Verification items for this drawing (mm, ordinates from the low corner). A direction names the side the tool comes from. Round coordinates to 2 decimals unless told otherwise and drop trailing zeros. Write each loop counter-clockwise with the first axis right and the second up, starting at its lowest first coordinate (ties: lowest second). Pieces come first, ordered by that corner, then holes.
Item 1: Cross-section at A-A (x = 29.5). Enter the section's corners in (y, z), then the cut area to 3 significant figures.
Item 2: Cross-section at B-B (y = 6.5). Enter the section's corners in (x, z), then the cut area to 3 significant figures.
Item 3: Access from +Z, -Z, +X, -X, +Y, -Y to the whole of each face (thin tool, end or side, straight path). Record for the marked faces 1, 2 and 3.
Item 4: Scan lines: probe 1 along Y at (x, z) = (4, 27.5) (3 decimals); probe 2 along Z at (x, y) = (8, 0.75); probe 3 along Y at (x, z) = (22, 2). Record each from-to range of solid material in increasing order.
Item 5: Cross-section at C-C (z = 26.5). Enter the section's corners in (x, y) (3 decimals).
Item 6: Cross-section at D-D (x = 9). Enter the section's corners in (y, z).
Item 7: Depth check by flat-ended pin: P1, Ø4, axis at x = 26.5, y = 4.5, coming from the +Z side; P2, Ø1.5, axis at y = 1.5, z = 18.5, coming from the +X side; P3, Ø3, axis at y = 6.5, z = 12.5, coming from the -X side. Enter the tip coordinate at first touch or a pass-through.
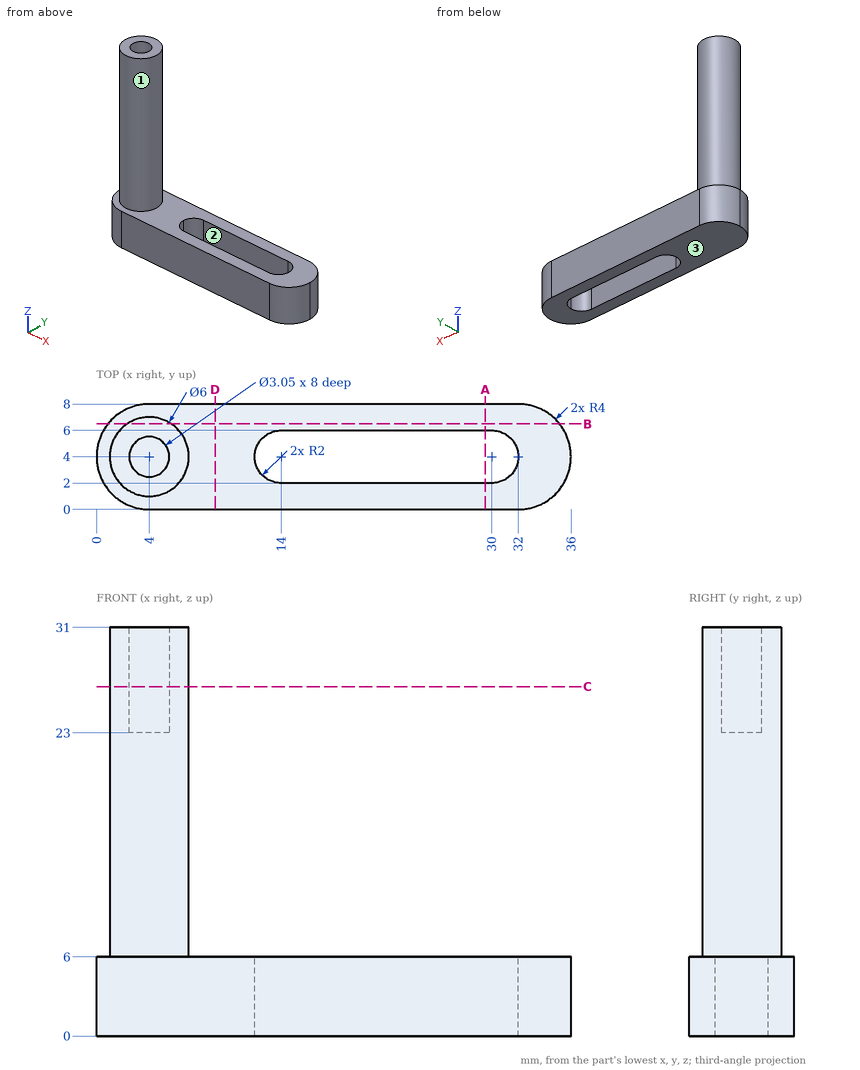
Resolved:
1. outline: (0, 0) - (2, 0) - (2, 6) - (0, 6) - close; (6, 0) - (8, 0) - (8, 6) - (6, 6) - close
1. area: 24.0 mm2
2. outline: (0.88, 0) - (35.12, 0) - (35.12, 6) - (5.66, 6) - (5.66, 31) - (2.34, 31) - (2.34, 6) - (0.88, 6) - close
2. area: 288 mm2
3. face 1: +Z
3. face 2: +Z, -Z
3. face 3: -Z, +X, -X, +Y, -Y
4. probe 1: y = 1 to 2.475, 5.525 to 7
4. probe 2: z = 0 to 6
4. probe 3: y = 0 to 2, 6 to 8
5. outline: circle Ø6 at (4, 4); hole circle Ø3.05 at (4, 4)
6. outline: (0, 0) - (8, 0) - (8, 6) - (0, 6) - close
7. P1: stops at z = 6
7. P2: stops at x = 6.44
7. P3: stops at x = 1.17
